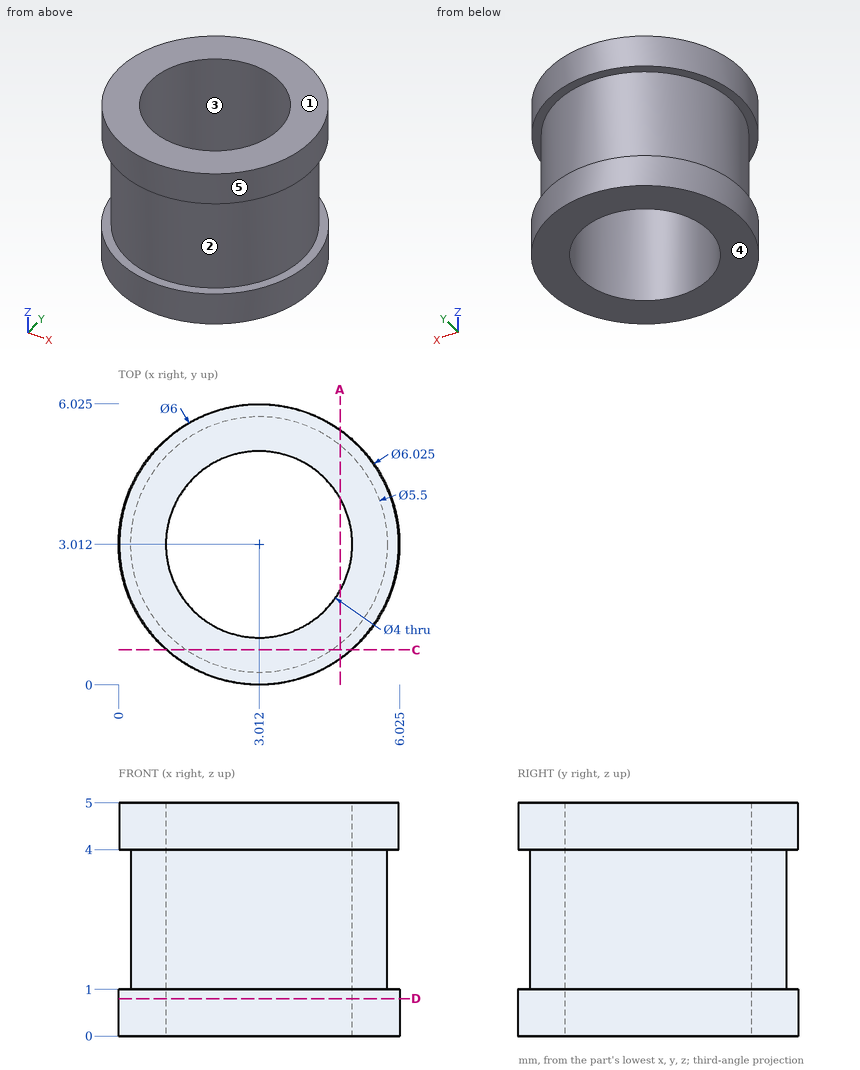
Could you check a few things on this drawing? It's one solid part, dimensions in mm from its lowest x, y, z. A direction names the side the tool comes from. Give positions to 0.01 mm unless a question says otherwise; leave off trailing zeros. Loops run counter-clockwise (first coordinate to the right, second up) from the corner with the lowest first, then second, coordinate; pieces in that order, holes last. Notation, with made-up numbers: (44.5, -10) -> (68.5, -10) arc R15 ccw to (68.5, 18) -> close; hole circle Ø7 at (88, 23.25). An arc over 180 degrees is marked (long way). Answer as CSV lines item,"result". Start each with the question number.
(1) If we section it at D-D on z = 0.8: Write out the boundary of the cut face in (x, y) (1 decimal).
(2) If we section it at A-A on x = 4.75: Write out the boundary of the cut face in (y, z), then the cut area to 3 significant figures.
(3) We'd pull the mould along Y, two halves only. Please class the marked faces 1, 2 and 3: released by +Y, released by -Y, zero draft, split by the parting line, or undercut.
(4) If we section it at C-C on y = 0.75: Write out the boundary of the cut face in (x, z) (1 decimal), then the cut area to 3 significant figures.
(5) I need wall thicknesses on probe 1 along Z at (x, y) = (1.5, 5.5); probe 2 along X at (y, z) = (3, 3.5); probe 3 along Y at (x, z) = (3.25, 0.85) (1 decimal). Which ranges of each line are inside material? Lowest first, please.
(6) Which directions (+Z, -Z, +X, -X, +Y, -Y) give clear straight access to the entire face, cutting with the end or side of a thin tool? Please do the marked faces 4 and 5.
Computed:
1,outline,"circle Ø6 at (3, 3); hole circle Ø4 at (3, 3)"
2,outline,"(0.55, 0) -> (2.02, 0) -> (2.02, 5) -> (0.57, 5) -> (0.57, 4) -> (0.88, 4) -> (0.88, 1) -> (0.55, 1) -> close; (4, 0) -> (5.47, 0) -> (5.47, 1) -> (5.14, 1) -> (5.14, 4) -> (5.46, 4) -> (5.46, 5) -> (4, 5) -> close"
2,area,"12.7 mm2"
3,face 1,"zero draft"
3,face 2,"split by the parting line"
3,face 3,"undercut"
4,outline,"(1, 0) -> (5, 0) -> (5, 1) -> (4.6, 1) -> (4.6, 4) -> (5, 4) -> (5, 5) -> (1, 5) -> (1, 4) -> (1.4, 4) -> (1.4, 1) -> (1, 1) -> close"
4,area,"17.3 mm2"
5,probe 1,"z = 0 to 1, 4 to 5"
5,probe 2,"x = 0.26 to 1.01, 5.01 to 5.76"
5,probe 3,"y = 0 to 1, 5 to 6"
6,face 4,"-Z, +X, -X, +Y, -Y"
6,face 5,"+Z"
